Check sheet for the modelled part. Datum: model origin and axes. Units: mm. Face numbers are marked on the shaded views. Round coordinates to 2 decimals unless told otherwise and drop trailing zeros. Write each loop counter-clockwise with the first axis right and the second up, starting at its lowest first coordinate (ties: lowest second). Pieces come first, ordered by that corner, then holes. Notation, with made-up numbers: (-20, 42.5) - (-13, 42.5) arc R26 cw to (-13, 78.5) - close; hole circle Ø7 at (23, -38). An arc over 180 degrees is marked (long way). Use one line per item in the form item = value. Start each with the question number.
1) Section check B-B (x = 33.5). Record the boundary of the cut face in (y, z).
2) Section check D-D (z = -2.25). Record the boundary of the cut face in (x, y).
3) Scan lines: probe 1 along Z at (x, y) = (12.7, 3.45) (3 decimals); probe 2 along X at (y, z) = (0.5, -9.5); probe 3 along X at (y, z) = (0.75, -8.25). Record each from-to range of solid material in increasing order.
4) Section check C-C (y = 3.25). Record the boundary of the cut face in (x, z) (3 decimals).
5) Gauge pin test, flat ends, axial feed: P1, Ø0.8, axis at y = 2.5, z = -14.5, coming from the -X side; P2, Ø1.5, axis at y = 3, z = -14.5, coming from the -X side; P3, Ø1.8, axis at x = 12.7, z = -8.255, coming from the -Y side (1 decimal); P4, Ø2, axis at x = 33.5, y = 4, coming from the +Z side. Record the tip position at first contact, or that the pin passes through.
6) Section check A-A (x = 12.7). Record the boundary of the cut face in (y, z) (3 decimals).
7) Draft check along X on the marked faces 1, 2, 3 and 4. Enter one of: +X half, -X half, draft (parallel to the pull), parting line (faces both ways), or undercut.
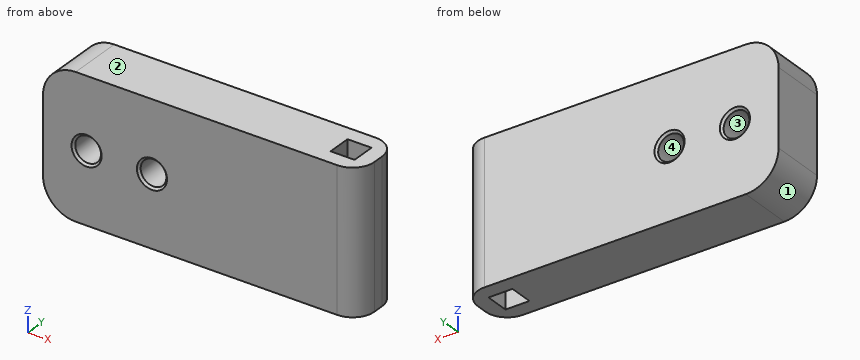
from build123d import *

# Parameters (mm, degrees)
SKETCH1_W             = 36.83
SKETCH1_H             = 16.51
BOSS_EXTRUDE1_DEPTH   = 6.35
F_3_0MM_DOWEL_HOLE1_D = 3
CHAMFER1_SIZE         = 0.254
FILLET2_R             = 3.81
SKETCH24_W            = 2.794
SKETCH24_H            = 2.794
CUT_EXTRUDE7_DEPTH    = 5.08
SKETCH25_W            = 2.794
SKETCH25_H            = 2.794
CUT_EXTRUDE8_DEPTH    = 5.08
FILLET7_R             = 2.54


with BuildPart() as part:
    # Sketch1 → Boss-Extrude1 (new body)
    with BuildSketch(Plane(origin=(0, 0, 0), x_dir=(1, 0, 0), z_dir=(0, 1, 0))):
        with Locations((18.415, 8.255)):
            Rectangle(SKETCH1_W, SKETCH1_H)
    extrude(amount=BOSS_EXTRUDE1_DEPTH)

    # Ø3.0mm Dowel Hole1 (through all)
    with Locations(Plane(origin=(0, 6.35, 0), x_dir=(1, 0, 0), z_dir=(0, 1, 0))):
        with Locations((5.08, 8.255), (12.7, 8.255)):
            Hole(F_3_0MM_DOWEL_HOLE1_D / 2)

    # Chamfer1
    chamfer1_edges = [part.edges().sort_by_distance(p)[0] for p in [
        (14.2, 6.35, -8.255),
        (14.2, 0, -8.255),
        (6.58, 6.35, -8.255),
        (6.58, 0, -8.255),
    ]]
    chamfer(chamfer1_edges, length=CHAMFER1_SIZE)

    # Fillet2
    fillet2_edges = [part.edges().sort_by_distance(p)[0] for p in [
        (0, 3.175, -16.51),
        (0, 3.175, 0),
    ]]
    fillet(fillet2_edges, radius=FILLET2_R)

    # Sketch24 → Cut-Extrude7 (cut)
    with BuildSketch(Plane.XY):
        with Locations((33.655, 3.175)):
            Rectangle(SKETCH24_W, SKETCH24_H)
    extrude(amount=-CUT_EXTRUDE7_DEPTH, mode=Mode.SUBTRACT)

    # Sketch25 → Cut-Extrude8 (cut)
    with BuildSketch(Plane(origin=(0, 0, -16.51), x_dir=(-1, 0, 0), z_dir=(0, 0, -1))):
        with Locations((-33.655, 3.175)):
            Rectangle(SKETCH25_W, SKETCH25_H)
    extrude(amount=-CUT_EXTRUDE8_DEPTH, mode=Mode.SUBTRACT)

    # Fillet7
    fillet7_edges = [part.edges().sort_by_distance(p)[0] for p in [
        (36.83, 6.35, -8.255),
        (36.83, 0, -8.255),
    ]]
    fillet(fillet7_edges, radius=FILLET7_R)


solid = part.part
Results are:
q1.outline = (0, -16.51) - (1.78, -16.51) - (1.78, -11.43) - (4.57, -11.43) - (4.57, -16.51) - (6.35, -16.51) - (6.35, 0) - (4.57, 0) - (4.57, -5.08) - (1.78, -5.08) - (1.78, 0) - (0, 0) - close
q2.outline = (0.33, 0) - (34.29, 0) arc R2.54 ccw to (36.83, 2.54) - (36.83, 3.81) arc R2.54 ccw to (34.29, 6.35) - (0.33, 6.35) - close; hole (32.26, 1.78) - (35.05, 1.78) - (35.05, 4.57) - (32.26, 4.57) - close
q3.probe_1 = -16.51 to -9.755, -6.755 to 0
q3.probe_2 = 0 to 4.24, 5.92 to 11.86, 13.54 to 35.8
q3.probe_3 = 0 to 3.58, 6.58 to 11.2, 14.2 to 36.09
q4.outline = (0, -12.7) arc R3.81 ccw to (3.81, -16.51) - (32.258, -16.51) - (32.258, -11.43) - (35.052, -11.43) - (35.052, -16.51) - (36.83, -16.51) - (36.83, 0) - (35.052, 0) - (35.052, -5.08) - (32.258, -5.08) - (32.258, 0) - (3.81, 0) arc R3.81 ccw to (0, -3.81) - close; hole circle Ø3 at (5.08, -8.255); hole circle Ø3 at (12.7, -8.255)
q5.P1 = 0.27
q5.P2 = 0.15
q5.P3 = through
q5.P4 = 0
q6.outline = (0, -16.51) - (6.35, -16.51) - (6.35, -10.009) - (6.096, -9.755) - (0.254, -9.755) - (0, -10.009) - close; (0, -6.501) - (0.254, -6.755) - (6.096, -6.755) - (6.35, -6.501) - (6.35, 0) - (0, 0) - close
q7.face_1 = -X half
q7.face_2 = draft
q7.face_3 = undercut
q7.face_4 = undercut
